```python
from build123d import *

# Parameters (mm, degrees)
SKETCH_1_R                   = 1.1
EXTRUDE_1_DEPTH              = 11
HOLE_WIZARD_M3_2_D           = 2.5
HOLE_WIZARD_M3_2_CSINK_D     = 3.05
HOLE_WIZARD_M3_2_CSINK_ANGLE = 90


with BuildPart() as part:
    # 草图1 → 凸台-拉伸1 (new body)
    with BuildSketch(Plane(origin=(0, 0, 0), x_dir=(1, 0, 0), z_dir=(0, 1, 0))):
        Polygon((1.231724884, -2.352910356), (2.653542583, -0.109750138), (1.421817699, 2.243160218), (-1.231724884, 2.352910356), (-2.653542583, 0.109750138), (-1.421817699, -2.243160218), align=None)
        Circle(SKETCH_1_R, mode=Mode.SUBTRACT)
    extrude(amount=EXTRUDE_1_DEPTH)

    # M3 螺纹孔2 (through all)
    with Locations(Plane(origin=(0, 11, 0), x_dir=(1, 0, 0), z_dir=(0, 1, 0))):
        with Locations((0, 0)):
            CounterSinkHole(HOLE_WIZARD_M3_2_D / 2, HOLE_WIZARD_M3_2_CSINK_D / 2, counter_sink_angle=HOLE_WIZARD_M3_2_CSINK_ANGLE)


solid = part.part
```
Geometry: final body of the model. Coordinates: model frame, mm. Round coordinates to 2 decimals unless told otherwise and drop trailing zeros. Write each loop counter-clockwise with the first axis right and the second up, starting at its lowest first coordinate (ties: lowest second). Pieces come first, ordered by that corner, then holes.
Item 1: Pin query (flat end, axial travel): P1, Ø1, axis at y = 6.5, z = 1.5, coming from the -X side. Return the tip coordinate at first contact, or that it passes through.
Item 2: Mould query, pull axis Z, two halves, no side actions, for faces 1 (the face through (0.27, 5.29, 1.22)), 2 (the face through (0, 11, 2)), 3 (the face through (-2.046, 5.423, 1.05)). Classes: +Z half, -Z half, draft (parallel to the pull), parting line (faces both ways), or undercut.
Item 3: Material intervals for L1, parallel to Z at x = 0, y = 3; L2, parallel to X at y = 4, z = 0.3; L3, parallel to X at y = 7.5, z = 0.15, sorted ascending.
Item 4: Section query D-D (x = 2.35). Return loops of the section in (y, z).
Item 5: Section query B-B (x = 0). Return loops of the section in (y, z) (3 decimals), plus the area to 3 significant figures.
Item 6: Section query A-A (y = 4). Return loops of the section in (x, z).
Item 7: Section query C-C (z = 0). Return loops of the section in (x, y) (3 decimals).
Completed:
1. P1: stops at x = -2.07
2. face 1: undercut
2. face 2: draft
2. face 3: +Z half
3. L1: z = -2.3 to -1.25, 1.25 to 2.3
3. L2: x = -2.44 to -1.21, 1.21 to 2.53
3. L3: x = -2.52 to -1.24, 1.24 to 2.63
4. outline: (0, -0.47) - (11, -0.47) - (11, 0.59) - (0, 0.59) - close
5. outline: (0, -2.302) - (11, -2.302) - (11, -1.525) - (10.725, -1.25) - (0, -1.25) - close; (0, 1.25) - (10.725, 1.25) - (11, 1.525) - (11, 2.302) - (0, 2.302) - close
5. area: 23.1 mm2
6. outline: (-2.65, -0.11) - (-1.23, -2.35) - (1.42, -2.24) - (2.65, 0.11) - (1.23, 2.35) - (-1.42, 2.24) - close; hole circle Ø2.5 at (0, 0)
7. outline: (-2.596, 0) - (-1.25, 0) - (-1.25, 10.725) - (-1.525, 11) - (-2.596, 11) - close; (1.25, 0) - (2.596, 0) - (2.596, 11) - (1.525, 11) - (1.25, 10.725) - close
